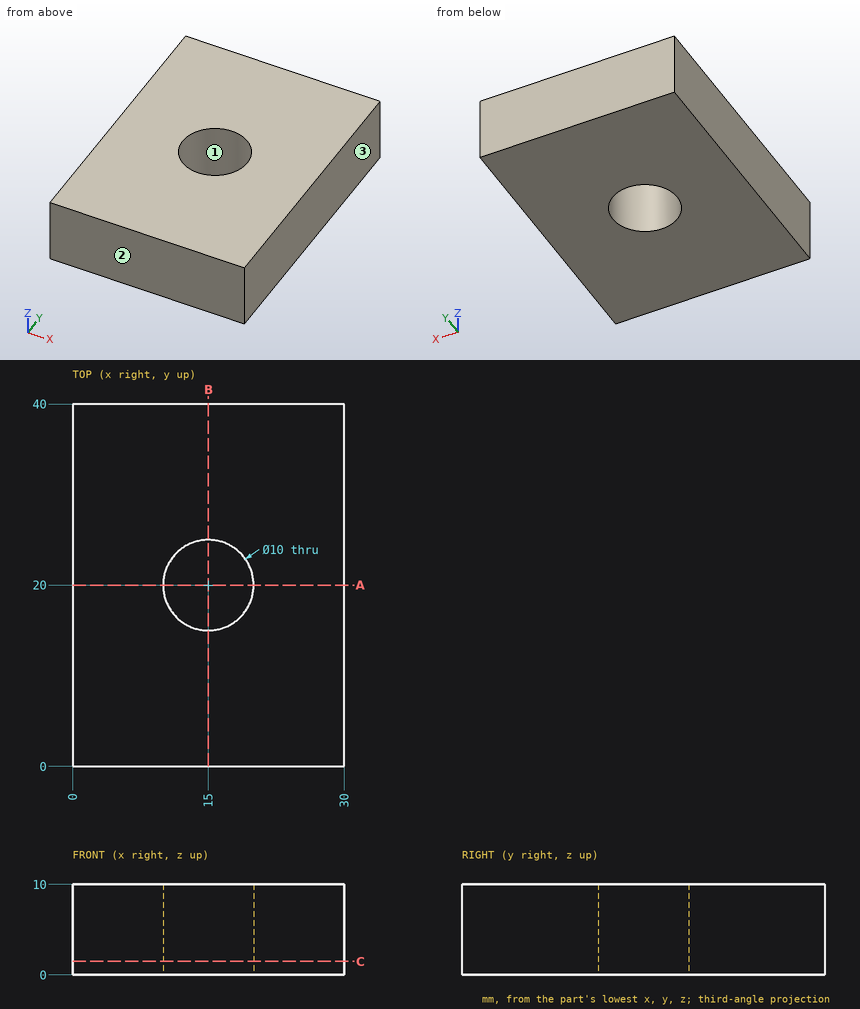
Study the drawing (mm; zero at the part's minimum x, y, z) and answer. Coordinates: 2 decimals unless noted, no trailing zeros. Loops run counter-clockwise (first coordinate to the right, second up) from the corner with the lowest first, then second, coordinate; pieces in that order, holes last. Notation, with made-up numbers: M 52.25,80 L 103.25,80 A17 ccw 103.25,108 Z; hole C 89.25,77 d11. An arc over 180 degrees is marked long. Answer in a Markdown table with one row per item. Add a question column.
1. Find section C-C, the plane z = 1.5. Write down the section's boundary in (x, y), then the cut area to 3 significant figures.
2. The mould has two halves that part along Y. Classify the marked faces 1, 2 and 3: pulls with the +Y half, pulls with the -Y half, needs draft (parallel to the pull), parting line crosses it, or undercut.
3. Find section B-B, the plane x = 15. Write down the section's boundary in (y, z).
4. Find section A-A, the plane y = 20. Write down the section's boundary in (x, z).
5. Consider L1, parallel to Y at x = 15, z = 5; L2, parallel to Y at x = 11, z = 1; L3, parallel to X at y = 22, z = 0.75. Determine where each line is inside the solid, lowest interval first.
Reported:
| question | item | result |
|---|---|---|
| 1 | outline | M 0,0 L 30,0 L 30,40 L 0,40 Z; hole C 15,20 d10 |
| 1 | area | 1,120 mm^2 |
| 2 | face 1 | undercut |
| 2 | face 2 | pulls with the -Y half |
| 2 | face 3 | needs draft |
| 3 | outline | M 0,0 L 15,0 L 15,10 L 0,10 Z; M 25,0 L 40,0 L 40,10 L 25,10 Z |
| 4 | outline | M 0,0 L 10,0 L 10,10 L 0,10 Z; M 20,0 L 30,0 L 30,10 L 20,10 Z |
| 5 | L1 | y = 0 to 15, 25 to 40 |
| 5 | L2 | y = 0 to 17, 23 to 40 |
| 5 | L3 | x = 0 to 10.42, 19.58 to 30 |
